```python
from build123d import *

# Parameters (mm, degrees)
SKETCH1_W           = 89
SKETCH1_H           = 9
BOSS_EXTRUDE1_DEPTH = 4
SKETCH2_R           = 1.75
CUT_EXTRUDE1_DEPTH  = 4
FILLET1_R           = 2
SKETCH4_W           = 28.175409777
SKETCH4_H           = 3
SKETCH4_W_2         = 27.315943202
CUT_EXTRUDE2_DEPTH  = 45.905456239
FILLET3_R           = 1


with BuildPart() as part:
    # Sketch1 → Boss-Extrude1 (new body)
    with BuildSketch(Plane(origin=(0, 0, 0), x_dir=(1, 0, 0), z_dir=(0, 1, 0))):
        Rectangle(SKETCH1_W, SKETCH1_H)
    extrude(amount=BOSS_EXTRUDE1_DEPTH)

    # Sketch2 → Cut-Extrude1 (cut)
    with BuildSketch(Plane(origin=(0, 4, 0), x_dir=(1, 0, 0), z_dir=(0, 1, 0))):
        with Locations(Location((-41, 0, 0), (0, 0, 270))):
            Circle(SKETCH2_R)
        with Locations(Location((41, 0, 0), (0, 0, 270))):
            Circle(SKETCH2_R)
    extrude(amount=-CUT_EXTRUDE1_DEPTH, mode=Mode.SUBTRACT)

    # Fillet1
    fillet1_edges = [part.edges().sort_by_distance(p)[0] for p in [
        (-44.5, 2, -4.5),
        (44.5, 2, -4.5),
        (44.5, 2, 4.5),
        (-44.5, 2, 4.5),
    ]]
    fillet(fillet1_edges, radius=FILLET1_R)

    # Sketch4 → Cut-Extrude2 (cut, through all)
    with BuildSketch(Plane(origin=(0, 4, 0), x_dir=(1, 0, 0), z_dir=(0, 1, 0))):
        with Locations((-19.087704888, 0)):
            Rectangle(SKETCH4_W, SKETCH4_H)
        with Locations((18.657971601, 0)):
            Rectangle(SKETCH4_W_2, SKETCH4_H)
    extrude(amount=-CUT_EXTRUDE2_DEPTH, mode=Mode.SUBTRACT)

    # Fillet3
    fillet3_edges = [part.edges().sort_by_distance(p)[0] for p in [
        (-33.175409777, 0, 0),
        (-33.175409777, 2, 1.5),
        (-19.087704888, 0, -1.5),
        (-33.175409777, 2, -1.5),
        (-5, 0, 0),
        (-5, 2, -1.5),
        (-19.087704888, 0, 1.5),
        (-5, 2, 1.5),
        (-33.175409777, 4, 0),
        (-19.087704888, 4, 1.5),
        (-5, 4, 0),
        (-19.087704888, 4, -1.5),
        (18.657971601, 0, 1.5),
        (32.315943202, 2, 1.5),
        (5, 0, 0),
        (5, 2, 1.5),
        (18.657971601, 0, -1.5),
        (5, 2, -1.5),
        (32.315943202, 0, 0),
        (32.315943202, 2, -1.5),
        (18.657971601, 4, 1.5),
        (32.315943202, 4, 0),
        (18.657971601, 4, -1.5),
        (5, 4, 0),
    ]]
    fillet(fillet3_edges, radius=FILLET3_R)


solid = part.part
```
Input: part model. Units: mm. Frame: model coordinates. A direction names the side the tool comes from. Round coordinates to 2 decimals unless told otherwise and drop trailing zeros. Loops run counter-clockwise (first coordinate to the right, second up) from the corner with the lowest first, then second, coordinate; pieces in that order, holes last. Notation, with made-up numbers: M 64,31.25 L 101,31.25 A18 ccw 101,36.25 Z; hole C 14,26 d11. An arc over 180 degrees is marked long. Answer in a Markdown table with one row per item. Add a question column.
1. Set-up query: faces 1 (the face through (18, 2, -1.5)), 2 (the face through (-1, 0, 0)). Return all of +Z, -Z, +X, -X, +Y, -Y with unobstructed straight access to the full face (end or side cutting, diameter ignored); none if empty.
2. Section A-A (x = -15). Output: boundary loops of the cut face in (y, z).
3. Mould query, pull axis X, two halves, no side actions, for faces 3 (the face through (18, 2, 1.5)), 4 (the face through (-44.5, 2, 0)), 5 (the face through (-1, 4, 0)), 6 (the face through (-19, 2, -1.5)). Classes: released by +X, released by -X, zero draft, split by the parting line, or undercut.
4. Section C-C (x = -41). Output: boundary loops of the cut face in (y, z).
5. Ray query, probe 1 along X at (y, z) = (2.85, 0); probe 2 along Z at (x, y) = (-29, 2.7); probe 3 along X at (y, z) = (1.15, -1). Return the intervals inside material, ascending.
6. Section B-B (y = 2.05). Output: boundary loops of the cut face in (x, z).
7. Contact query for a flat-ended pin moving along its axis: pin 1 (2 mm diameter, centred on x = 41, z = 0, fed in from -Y). Output: stop coordinate, or through.
Values follow:
| question | item | result |
|---|---|---|
| 1 | face 1 | +Y, -Y |
| 1 | face 2 | +Z, -Z, +X, -X, -Y |
| 2 | outline | M 0,-4.5 L 4,-4.5 L 4,-2.5 A1 ccw 3,-1.5 L 1,-1.5 A1 ccw 0,-2.5 Z; M 0,2.5 A1 ccw 1,1.5 L 3,1.5 A1 ccw 4,2.5 L 4,4.5 L 0,4.5 Z |
| 3 | face 3 | undercut |
| 3 | face 4 | released by -X |
| 3 | face 5 | zero draft |
| 3 | face 6 | undercut |
| 4 | outline | M 0,-4.5 L 4,-4.5 L 4,-1.75 L 0,-1.75 Z; M 0,1.75 L 4,1.75 L 4,4.5 L 0,4.5 Z |
| 5 | probe 1 | -44.5 to -42.75, -39.25 to -33.18, -5 to 5, 32.32 to 39.25, 42.75 to 44.5 |
| 5 | probe 2 | -4.5 to -1.5, 1.5 to 4.5 |
| 5 | probe 3 | -44.5 to -42.44, -39.56 to -33.04, -5.13 to 5.13, 32.18 to 39.56, 42.44 to 44.5 |
| 6 | outline | M -44.5,-2.5 A2 ccw -42.5,-4.5 L 42.5,-4.5 A2 ccw 44.5,-2.5 L 44.5,2.5 A2 ccw 42.5,4.5 L -42.5,4.5 A2 ccw -44.5,2.5 Z; hole C -41,0 d3.5; hole M -33.18,-0.5 A1 ccw -32.18,-1.5 L -6,-1.5 A1 ccw -5,-0.5 L -5,0.5 A1 ccw -6,1.5 L -32.18,1.5 A1 ccw -33.18,0.5 Z; hole M 5,-0.5 A1 ccw 6,-1.5 L 31.32,-1.5 A1 ccw 32.32,-0.5 L 32.32,0.5 A1 ccw 31.32,1.5 L 6,1.5 A1 ccw 5,0.5 Z; hole C 41,0 d3.5 |
| 7 | pin 1 | through |
